The drawing under review shows one solid part. Ordinate dimensions are in mm from its lowest x, y, z. A direction names the side the tool comes from. Coordinates: 2 decimals unless noted, no trailing zeros. Order: outer loops, then holes, each group sorted by start corner. A loop starts at its lowest first (then second) coordinate and runs counter-clockwise, first axis right, second up.
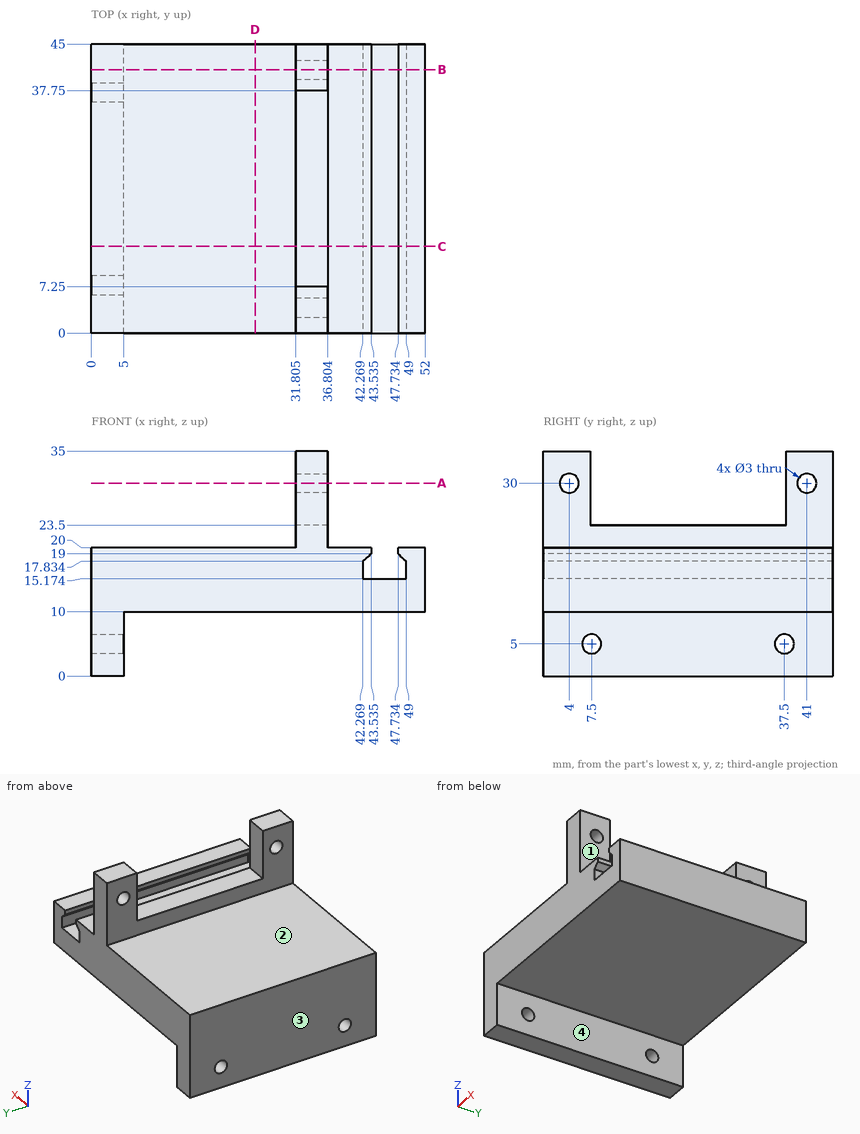
1. Clearance check with flat-ended pins moving along their axes: pin 1 Ø6 at (x, y) = (11.5, 24.5) entering from +Z; pin 2 Ø1 at (x, y) = (35, 7) entering from -Z; pin 3 Ø8 at (x, z) = (32, 16.5) entering from -Y; pin 4 Ø3 at (y, z) = (14, 7.5) entering from +X. State where each tip first meets the part, or that it passes through.
Answer below:
pin 1: stops at z = 20
pin 2: stops at z = 10
pin 3: stops at y = 0
pin 4: stops at x = 5
2. Take a section at D-D, the plane x = 25.5. Give the boundary of the cut face in (y, z).
Answer below:
outline: (0, 10) - (45, 10) - (45, 20) - (0, 20) - close
3. Machinability: for the marked faces 1, 2, 3 and 4, which of the approach directions +Z, -Z, +X, -X, +Y, -Y give a long, thin tool a straight path to every point of the face, cutting with its end or side? Answer none if there is none.
Answer below:
face 1: +Z, +X, +Y, -Y
face 2: +Z, -X, +Y, -Y
face 3: +Z, -Z, -X, +Y, -Y
face 4: -Z, +X, +Y, -Y
4. Take a section at C-C, the plane y = 13.5. Give the boundary of the cut face in (x, z) (1 decimal), plus the area to 3 significant figures.
Answer below:
outline: (0, 0) - (5, 0) - (5, 10) - (52, 10) - (52, 20) - (47.7, 20) - (47.7, 19) - (49, 17.8) - (49, 15.2) - (42.3, 15.2) - (42.3, 17.8) - (43.5, 19) - (43.5, 20) - (36.8, 20) - (36.8, 23.5) - (31.8, 23.5) - (31.8, 20) - (0, 20) - close
area: 559 mm2
5. Take a section at B-B, the plane y = 41. Give the boundary of the cut face in (x, z) (1 decimal).
Answer below:
outline: (0, 0) - (5, 0) - (5, 10) - (52, 10) - (52, 20) - (47.7, 20) - (47.7, 19) - (49, 17.8) - (49, 15.2) - (42.3, 15.2) - (42.3, 17.8) - (43.5, 19) - (43.5, 20) - (36.8, 20) - (36.8, 28.5) - (31.8, 28.5) - (31.8, 20) - (0, 20) - close; (31.8, 31.5) - (36.8, 31.5) - (36.8, 35) - (31.8, 35) - close
6. To check wall thickness, follow L1, parallel to Y at x = 2.6, z = 5; L2, parallel to Y at x = 34.1, z = 30; L3, parallel to Z at x = 14, y = 35. State the ranges of each line that lie inside material, in increasing order.
Answer below:
L1: y = 0 to 6, 9 to 36, 39 to 45
L2: y = 0 to 2.5, 5.5 to 7.25, 37.75 to 39.5, 42.5 to 45
L3: z = 10 to 20
7. Take a section at A-A, the plane z = 30. Give the number of separate pieces and of enclosed holes in the cut face.
Answer below:
separate pieces: 4
enclosed holes: 0
